Input: dimensioned drawing with shaded views. Units: mm. Origin: part minimum x, y, z. Coordinates: 2 decimals unless noted, no trailing zeros. Order: outer loops, then holes, each group sorted by start corner. A loop starts at its lowest first (then second) coordinate and runs counter-clockwise, first axis right, second up. Notation, with made-up numbers: (7, 7) -> (34, 7) arc R15 cw to (34, 33) -> close; hole circle Ø8 at (30.25, -28). An arc over 180 degrees is marked (long way). Answer in a Markdown table with one row per item. Add a question column.
1) Section query A-A on x = 30. Return the cut outline in (y, z), then the cut area to 3 significant figures.
2) Section query D-D on y = 55. Return the cut outline in (x, z), then the cut area to 3 significant figures.
3) Contact query for a flat-ended pin moving along its axis: P1, Ø6.5, axis at x = 30, y = 55, coming from the -Z side. Output: stop coordinate, or through.
4) Ray query, line 1 (Y direction, x = 30, z = 0.75); line 2 (Y direction, x = 28, z = 0.15); line 3 (Y direction, x = 48, z = 0.85). Return the intervals inside material, ascending. Write a range as from..to.
5) Section query C-C on x = 12. Return the cut outline in (y, z).
6) Section query B-B on y = 10. Return the cut outline in (x, z), then the cut area to 3 significant figures.
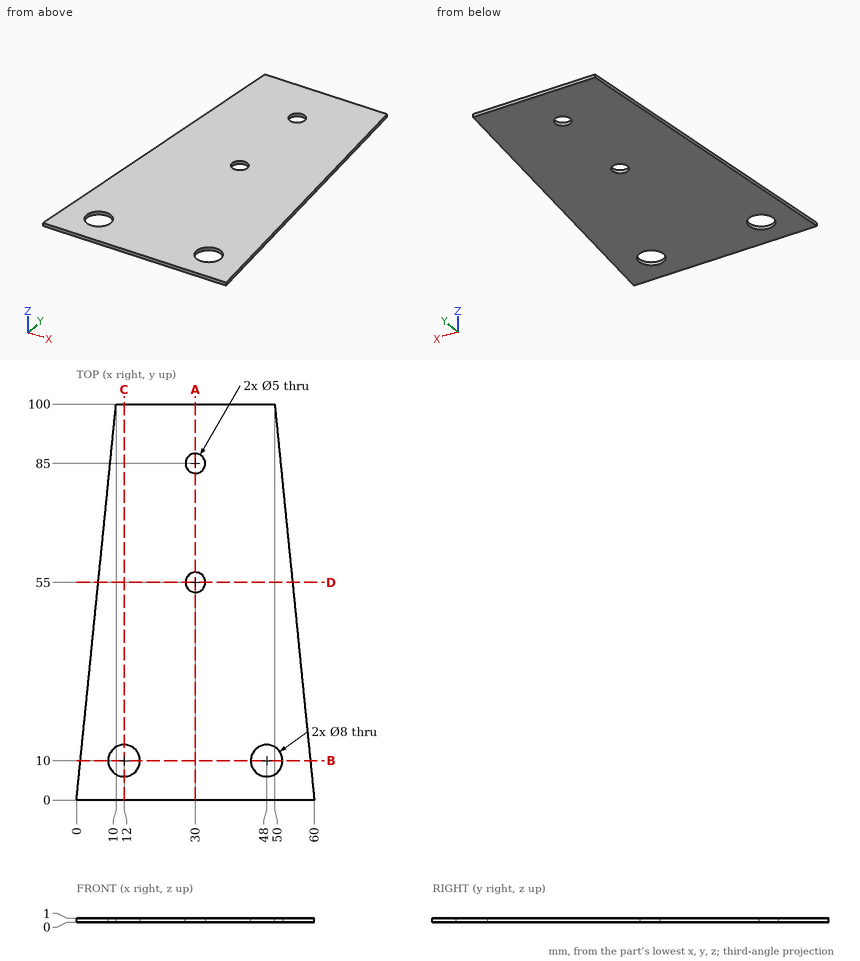
Result:
| question | item | result |
|---|---|---|
| 1 | outline | (0, 0) -> (52.5, 0) -> (52.5, 1) -> (0, 1) -> close; (57.5, 0) -> (82.5, 0) -> (82.5, 1) -> (57.5, 1) -> close; (87.5, 0) -> (100, 0) -> (100, 1) -> (87.5, 1) -> close |
| 1 | area | 90.0 mm2 |
| 2 | outline | (5.5, 0) -> (27.5, 0) -> (27.5, 1) -> (5.5, 1) -> close; (32.5, 0) -> (54.5, 0) -> (54.5, 1) -> (32.5, 1) -> close |
| 2 | area | 44.0 mm2 |
| 3 | P1 | z = 0 |
| 4 | line 1 | 0..52.5, 57.5..82.5, 87.5..100 |
| 4 | line 2 | 0..53.5, 56.5..83.5, 86.5..100 |
| 4 | line 3 | 0..6, 14..100 |
| 5 | outline | (0, 0) -> (6, 0) -> (6, 1) -> (0, 1) -> close; (14, 0) -> (100, 0) -> (100, 1) -> (14, 1) -> close |
| 6 | outline | (1, 0) -> (8, 0) -> (8, 1) -> (1, 1) -> close; (16, 0) -> (44, 0) -> (44, 1) -> (16, 1) -> close; (52, 0) -> (59, 0) -> (59, 1) -> (52, 1) -> close |
| 6 | area | 42.0 mm2 |
